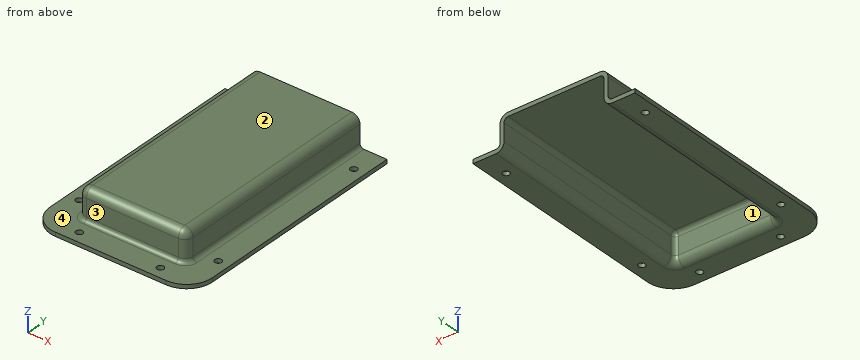
Autodesk Inventor part; units mm, degrees
ref_plane "YZ Plane" through (0, 0, 0) normal (1, 0, 0) x (0, 1, 0)
ref_plane "XZ Plane" through (0, 0, 0) normal (0, 1, 0) x (-1, 0, 0)
ref_plane "XY Plane" through (0, 0, 0) normal (0, 0, 1) x (1, 0, 0)
sketch "Sketch1" plane through (0, 0, 0) normal (0, 0, 1) x (1, 0, 0)
  line L0 (-25.4, 50.8) -> (25.4, 50.8)
  line L1 (25.4, 50.8) -> (25.4, -50.8)
  line L2 (25.4, -50.8) -> (-25.4, -50.8)
  line L3 (-25.4, -50.8) -> (-25.4, 50.8)
  point P0 (0, 0)
  point P1 (0, 50.8)
  point P2 (-25.4, 0)
  dimension "Width" = 50.8
  dimension "Height" = 101.6
extrude "Extrusion1" add sketch "Sketch1" along normal blind 15.875
shell "Shell1" thickness 1.905 removed faces 2 at (-8.4667, 50.8, 5.2917) at (-8.4667, 16.9333, 0)
sketch "Sketch2" plane through (0, 0, 0) normal (0, 0, -1) x (-1, 0, 0)
  line L0 (-25.4, 50.8) -> (-25.4, -50.8)
  line L1 (25.4, -50.8) -> (25.4, 50.8)
  line L2 (-25.4, -50.8) -> (25.4, -50.8)
  line L3 (25.4, 50.8) -> (38.1, 50.8)
  line L4 (38.1, 50.8) -> (38.1, -51.435)
  arc A0 (26.035, -63.5) -> (38.1, -51.435) centre (26.035, -51.435) ccw
  line L5 (26.035, -63.5) -> (-26.035, -63.5)
  arc A1 (-38.1, -51.435) -> (-26.035, -63.5) centre (-26.035, -51.435) ccw
  line L6 (-38.1, -51.435) -> (-38.1, 50.8)
  line L7 (-38.1, 50.8) -> (-25.4, 50.8)
  dimension "d5" = 12.7
  dimension "d6" = 12.7
  dimension "d7" = 12.065
extrude "Extrusion2" add sketch "Sketch2" against normal blind 1.905
fillet "Fillet1" radius 1.905 8 edges at (23.495, 0.9525, 13.97) (0, -48.895, 13.97) (23.495, -48.895, 6.985) (-23.495, -48.895, 6.985) (-23.495, 0.9525, 13.97) (-25.4, 0, 1.905) (0, -50.8, 1.905) (25.4, 0, 1.905)
fillet "Fillet1" radius 3.81 8 edges at (0, -50.8, 15.875) (25.4, 0, 15.875) (-25.4, 0, 15.875) (-25.4, -50.8, 8.89) (25.4, -50.8, 8.89) (-23.495, 0.9525, 0) (0, -48.895, 0) (23.495, 0.9525, 0)
sketch "Sketch3" plane through (0, 0, 0) normal (0, 0, -1) x (-1, 0, 0)
  line L0 (-27.305, 50.8) -> (-38.1, 50.8)
  arc A0 (-38.1, -51.435) -> (-26.035, -63.5) centre (-26.035, -51.435) ccw
  line L1 (-38.1, -51.435) -> (-38.1, 50.8)
  line L2 (26.035, -63.5) -> (-26.035, -63.5)
  line L3 (0, -63.5) -> (0, -52.705) construction
  line L4 (-21.59, -52.705) -> (21.59, -52.705) construction
  line L5 (0, -89.3585) -> (0, 74.1597) construction
  point P0 (-32.7025, 38.1)
  point P1 (-32.7025, -41.275)
  point P2 (-19.05, -58.1025)
  point P3 (-32.7025, 50.8)
  point P4 (-32.7025, 50.8)
  point P5 (0, -58.1025)
  point P6 (32.7025, 38.1)
  point P7 (32.7025, -41.275)
  point P8 (19.05, -58.1025)
  dimension "d13" = 19.05
  dimension "d14" = 22.225
  dimension "d15" = 12.7
hole "Hole1" at (32.7025, 38.1, 0) at (32.7025, -41.275, 0) at (19.05, -58.1025, 0) at (-32.7025, 38.1, 0) at (-32.7025, -41.275, 0) at (-19.05, -58.1025, 0) direction (0, 0, 1) diameter 3.175 end through all
properties part number "M178-4001-03" material "Plastic, Clear"
Input: part model. Units: mm. Frame: model coordinates. Face numbers are marked on the shaded views. A direction names the side the tool comes from. Give positions to 0.01 mm unless a question says otherwise; leave off trailing zeros. Write each loop counter-clockwise with the first axis right and the second up, starting at its lowest first coordinate (ties: lowest second). Pieces come first, ordered by that corner, then holes. Notation, with made-up numbers: M 67.25,-39 L 81.25,-39 A28 ccw 81.25,-12 Z; hole C -14.75,83.25 d7. An arc over 180 degrees is marked long. Use one line per item in the form item = value.
1. Cut plane D-D on x = -10. Return loops of the section in (y, z) (3 decimals), and give its area (3 significant figures).
Outcome:
outline = M -63.5,0 L -52.705,0 A3.81 ccw -48.895,3.81 L -48.895,12.065 A1.905 cw -46.99,13.97 L 50.8,13.97 L 50.8,15.875 L -46.99,15.875 A3.81 ccw -50.8,12.065 L -50.8,3.81 A1.905 cw -52.705,1.905 L -63.5,1.905 Z
area = 240 mm²
2. Ray query, L1, parallel to X at y = 34, z = 9.25 (3 decimals); L2, parallel to Z at x = -9.5, y = -19 (3 decimals); L3, parallel to Z at x = 33.5, y = -53 (3 decimals). Return the intervals inside material, ascending.
Outcome:
L1 = -25.4 to -23.495, 23.495 to 25.4
L2 = 13.97 to 15.875
L3 = 0 to 1.905
3. Reachability of the marked faces 1, 2, 3 and 4 from +Z, -Z, +X, -X, +Y, -Y: full face, straight path, thin tool, end or side. Return the list, or none.
Outcome:
face_1 = -Z, +Y
face_2 = +Z, +X, -X, +Y, -Y
face_3 = +Z, +X, -X, -Y
face_4 = +Z, -Y
4. Cut plane B-B on x = -19.05. Return loops of the section in (y, z) (3 decimals), and give its area (3 significant figures).
Outcome:
outline = M -63.5,0 L -59.69,0 L -59.69,1.905 L -63.5,1.905 Z; M -56.515,0 L -52.705,0 A3.81 ccw -48.895,3.81 L -48.895,12.065 A1.905 cw -46.99,13.97 L 50.8,13.97 L 50.8,15.875 L -46.99,15.875 A3.81 ccw -50.8,12.065 L -50.8,3.81 A1.905 cw -52.705,1.905 L -56.515,1.905 Z
area = 234 mm²
5. Cut plane A-A on y = 38.1. Return loops of the section in (x, z) (3 decimals), and give its area (3 significant figures).
Outcome:
outline = M -38.1,0 L -34.29,0 L -34.29,1.905 L -38.1,1.905 Z; M -31.115,0 L -27.305,0 A3.81 ccw -23.495,3.81 L -23.495,12.065 A1.905 cw -21.59,13.97 L 21.59,13.97 A1.905 cw 23.495,12.065 L 23.495,3.81 A3.81 ccw 27.305,0 L 31.115,0 L 31.115,1.905 L 27.305,1.905 A1.905 cw 25.4,3.81 L 25.4,12.065 A3.81 ccw 21.59,15.875 L -21.59,15.875 A3.81 ccw -25.4,12.065 L -25.4,3.81 A1.905 cw -27.305,1.905 L -31.115,1.905 Z; M 34.29,0 L 38.1,0 L 38.1,1.905 L 34.29,1.905 Z
area = 177 mm²
6. First-contact query: P1, Ø2.5, axis at y = -21, z = 7, coming from the +X side; P2, Ø4, axis at x = 1, z = 7, coming from the +Y side (3 decimals); P3, Ø3, axis at x = 19.05, y = -58.1, coming from the +Z side; P4, Ø2.5, axis at y = -2, z = 9, coming from the -X side. Flat tips, straight axial feed; report the tip coordinate or a pass-through.
Outcome:
P1 = 25.4
P2 = -48.895
P3 = through
P4 = -25.4
7. Cut plane C-C on y = 15. Return loops of the section in (x, z) (3 decimals), and give its area (3 significant figures).
Outcome:
outline = M -38.1,0 L -27.305,0 A3.81 ccw -23.495,3.81 L -23.495,12.065 A1.905 cw -21.59,13.97 L 21.59,13.97 A1.905 cw 23.495,12.065 L 23.495,3.81 A3.81 ccw 27.305,0 L 38.1,0 L 38.1,1.905 L 27.305,1.905 A1.905 cw 25.4,3.81 L 25.4,12.065 A3.81 ccw 21.59,15.875 L -21.59,15.875 A3.81 ccw -25.4,12.065 L -25.4,3.81 A1.905 cw -27.305,1.905 L -38.1,1.905 Z
area = 189 mm²
